```python
from build123d import *

# Parameters (mm, degrees)
SKETCH1_W           = 31.75
SKETCH1_H           = 31.75
BOSS_EXTRUDE1_DEPTH = 1828.8
SKETCH2_W           = 19.05
SKETCH2_H           = 19.05
CUT_EXTRUDE1_DEPTH  = 1829.8
SKETCH3_R           = 3.175
CUT_EXTRUDE2_DEPTH  = 32.75
SKETCH4_R           = 3.175
CUT_EXTRUDE3_DEPTH  = 32.75


with BuildPart() as part:
    # Sketch1 → Boss-Extrude1 (new body)
    with BuildSketch(Plane(origin=(0, 0, 0), x_dir=(1, 0, 0), z_dir=(0, 1, 0))):
        with Locations((15.875, 15.875)):
            Rectangle(SKETCH1_W, SKETCH1_H)
    extrude(amount=BOSS_EXTRUDE1_DEPTH)

    # Sketch2 → Cut-Extrude1 (cut, through all)
    with BuildSketch(Plane(origin=(0, 1828.8, 0), x_dir=(1, 0, 0), z_dir=(0, 1, 0))):
        with Locations((15.875, 15.875)):
            Rectangle(SKETCH2_W, SKETCH2_H)
    extrude(amount=-CUT_EXTRUDE1_DEPTH, mode=Mode.SUBTRACT)

    # Sketch3 → Cut-Extrude2 (cut, through all)
    with BuildSketch(Plane(origin=(31.75, 0, 0), x_dir=(0, 0, -1), z_dir=(1, 0, 0))):
        with Locations((15.875, 1727.2)):
            Circle(SKETCH3_R)
    extrude(amount=-CUT_EXTRUDE2_DEPTH, mode=Mode.SUBTRACT)

    # Sketch4 → Cut-Extrude3 (cut, through all)
    with BuildSketch(Plane(origin=(31.75, 0, 0), x_dir=(0, 0, -1), z_dir=(1, 0, 0))):
        with Locations((15.875, 1524)):
            Circle(SKETCH4_R)
        with Locations((15.875, 1219.2)):
            Circle(SKETCH4_R)
        with Locations((15.875, 914.4)):
            Circle(SKETCH4_R)
        with Locations((15.875, 609.6)):
            Circle(SKETCH4_R)
        with Locations((15.875, 406.4)):
            Circle(SKETCH4_R)
    extrude(amount=-CUT_EXTRUDE3_DEPTH, mode=Mode.SUBTRACT)


solid = part.part
```
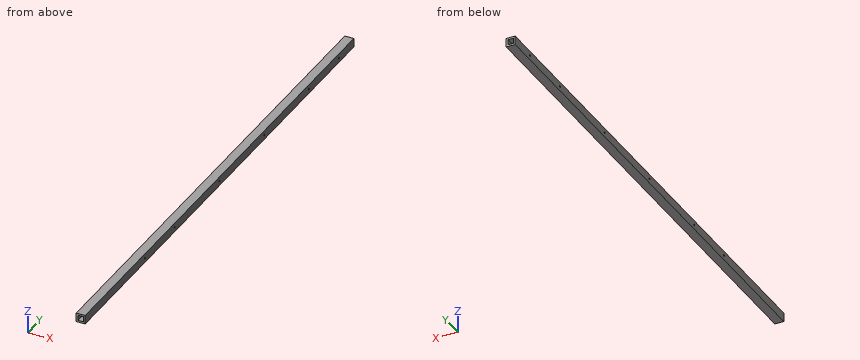
Can you work these out from the model? Positions are in its coordinate system, mm. Round coordinates to 2 decimals unless told otherwise and drop trailing zeros. Loops run counter-clockwise (first coordinate to the right, second up) from the corner with the lowest first, then second, coordinate; pieces in that order, holes last. Notation, with made-up numbers: (21, 77.5) -> (41, 77.5) arc R17 ccw to (41, 81.5) -> close; hole circle Ø1 at (28, 4). An arc over 180 degrees is marked (long way). One line per item, written item: value. Start each with the question number.
1. If we section it at A-A, the plane x = 19.5: Write out the boundary of the cut face in (y, z), then the cut area to 3 significant figures.
2. If I drill on probe 1 along Z at (x, y) = (27, 914); probe 2 along X at (y, z) = (730, -10.5); probe 3 along Z at (x, y) = (20, 1423), over which ranges is the centre line in solid material (lowest first)?
3. For pin 1 (10 mm diameter, centred on y = 1727.2, z = -15.875, fed in from -X), with a flat end and sliding along its axis, tell me the tip position at first contact or that it passes through.
4. If we section it at B-B, the plane y = 1457.5: Write out the boundary of the cut face in (x, z), then the cut area to 3 significant figures.
Calculated:
1. outline: (0, -31.75) -> (1828.8, -31.75) -> (1828.8, -25.4) -> (0, -25.4) -> close; (0, -6.35) -> (1828.8, -6.35) -> (1828.8, 0) -> (0, 0) -> close
1. area: 23,200 mm²
2. probe 1: z = -31.75 to -19.02, -12.73 to 0
2. probe 2: x = 0 to 6.35, 25.4 to 31.75
2. probe 3: z = -31.75 to -25.4, -6.35 to 0
3. pin 1: stops at x = 0
4. outline: (0, -31.75) -> (31.75, -31.75) -> (31.75, 0) -> (0, 0) -> close; hole (6.35, -25.4) -> (25.4, -25.4) -> (25.4, -6.35) -> (6.35, -6.35) -> close
4. area: 645 mm²
